from build123d import *

# Parameters (mm, degrees)
SKETCH1_W                          = 12.954
SKETCH1_H                          = 29.972
EXTRUDE1_DEPTH                     = 6.477
SKETCH2_W                          = 6.35
SKETCH2_H                          = 17.526
EXTRUDE2_DEPTH                     = 13.954
SKETCH5_R                          = 3.175
EXTRUDE3_DEPTH                     = 13.954
F_5_16_24_TAPPED_HOLE1_D           = 7.9375
F_5_16_24_TAPPED_HOLE1_DEPTH       = 12.446
F_5_16_24_TAPPED_HOLE1_CSINK_D     = 9.2075
F_5_16_24_TAPPED_HOLE1_CSINK_ANGLE = 90


with BuildPart() as part:
    # Sketch1 → Extrude1 (new body, symmetric)
    with BuildSketch(Plane(origin=(0, 0, 0), x_dir=(1, 0, 0), z_dir=(0, 1, 0))):
        Rectangle(SKETCH1_W, SKETCH1_H)
    extrude(amount=EXTRUDE1_DEPTH, both=True)

    # Sketch2 → Extrude2 (cut, through all)
    with BuildSketch(Plane(origin=(0, 6.477, 0), x_dir=(1, 0, 0), z_dir=(0, 1, 0))):
        with Locations((0, 6.223)):
            Rectangle(SKETCH2_W, SKETCH2_H)
    extrude(amount=-EXTRUDE2_DEPTH, mode=Mode.SUBTRACT)

    # Sketch5 → Extrude3 (cut, through all)
    with BuildSketch(Plane(origin=(6.477, 0, 0), x_dir=(0, 0, -1), z_dir=(1, 0, 0))):
        with Locations((8.89, 0)):
            Circle(SKETCH5_R)
    extrude(amount=-EXTRUDE3_DEPTH, mode=Mode.SUBTRACT)

    # 5/16-24 Tapped Hole1
    with Locations(Plane.XY.offset(14.986)):
        with Locations((0, 0)):
            CounterSinkHole(F_5_16_24_TAPPED_HOLE1_D / 2, F_5_16_24_TAPPED_HOLE1_CSINK_D / 2, depth=F_5_16_24_TAPPED_HOLE1_DEPTH, counter_sink_angle=F_5_16_24_TAPPED_HOLE1_CSINK_ANGLE)


solid = part.part
For this review, take the finished solid that the model builds, in its own axes (mm). A direction names the side the tool comes from. Give positions to 0.01 mm unless a question says otherwise; leave off trailing zeros. Loops run counter-clockwise (first coordinate to the right, second up) from the corner with the lowest first, then second, coordinate; pieces in that order, holes last.
Item 1: Take a section at C-C, the plane x = 0. State the section outline as (y, z) points, and give its area (3 significant figures).
Item 2: Tool access review of faces 1 (the flat face through (0, 5, 2.54)), 2 (the cylindrical face through (0.86, -3.874, 8.363)), 3 (the flat face through (-5, 0, -14.986)): name each direction out of +Z, -Z, +X, -X, +Y, -Y from which nothing blocks a thin tool from reaching the whole face with its end or side.
Item 3: Take a section at B-B, the plane z = -8.89. State the section outline as (x, y) points (3 decimals).
Item 4: Take a section at A-A, the plane y = 0. State the section outline as (x, z) points (3 decimals).
Item 5: For line 1 along X through (y, z) = (-5.5, -5.75) (3 decimals); line 2 along Z through (x, y) = (1, 4.5), list the stretches that pass through material, from the lowest coordinate up.
Item 6: Draft analysis for pull direction X (two halves, no side actions). For faces 4 (the flat face through (-3.175, 0, -4)), 5 (the flat face through (-6.477, 0, 0)), 6 (the flat face through (0, -5, 2.54)), 7 (the flat face through (-4, 3, 14.986)), state which applies: +X half, -X half, draft (parallel to the pull), parting line (faces both ways), or undercut.
Item 7: Insertion check: pin 1 (1.2 mm diameter, centred on x = 1, y = -4.5, fed in from -Z); pin 2 (4 mm diameter, centred on y = 0, z = -8.89, fed in from -X) (1 decimal); pin 3 (4 mm diameter, centred on x = -1.5, y = 0, fed in from +Z). Each pin has a flat end and moves straight along its axis. Give the tip position at first contact, or say it passes through.
Item 8: Take a section at D-D, the plane z = 1.5. State the section outline as (x, y) points (3 decimals), and give its area (3 significant figures).
Calculated:
1. outline: (-6.48, 2.54) - (-3.97, 2.54) - (-3.97, 14.35) - (-4.6, 14.99) - (-6.48, 14.99) - close; (3.97, 2.54) - (6.48, 2.54) - (6.48, 14.99) - (4.6, 14.99) - (3.97, 14.35) - close
1. area: 62.0 mm2
2. face 1: -Z, +Y, -Y
2. face 2: +Z
2. face 3: -Z, +X, -X, +Y, -Y
3. outline: (-6.477, -6.477) - (-3.175, -6.477) - (-3.175, -3.175) - (-6.477, -3.175) - close; (-6.477, 3.175) - (-3.175, 3.175) - (-3.175, 6.477) - (-6.477, 6.477) - close; (3.175, -6.477) - (6.477, -6.477) - (6.477, -3.175) - (3.175, -3.175) - close; (3.175, 3.175) - (6.477, 3.175) - (6.477, 6.477) - (3.175, 6.477) - close
4. outline: (-6.477, -14.986) - (-3.175, -14.986) - (-3.175, -12.065) - (-6.477, -12.065) - close; (-6.477, -5.715) - (-3.175, -5.715) - (-3.175, 2.54) - (-3.969, 2.54) - (-3.969, 14.351) - (-4.604, 14.986) - (-6.477, 14.986) - close; (3.175, -14.986) - (6.477, -14.986) - (6.477, -12.065) - (3.175, -12.065) - close; (3.175, -5.715) - (6.477, -5.715) - (6.477, 14.986) - (4.604, 14.986) - (3.969, 14.351) - (3.969, 2.54) - (3.175, 2.54) - close
5. line 1: x = -6.477 to -3.175, 3.175 to 6.477
5. line 2: z = 2.54 to 14.99
6. face 4: undercut
6. face 5: -X half
6. face 6: undercut
6. face 7: draft
7. pin 1: stops at z = 2.54
7. pin 2: passes through
7. pin 3: stops at z = 2.54
8. outline: (-6.477, -6.477) - (-3.175, -6.477) - (-3.175, 6.477) - (-6.477, 6.477) - close; (3.175, -6.477) - (6.477, -6.477) - (6.477, 6.477) - (3.175, 6.477) - close
8. area: 85.5 mm2
